Geometry: see drawing. Coordinates: mm, zero at the bounding-box minimum. A direction names the side the tool comes from. Round coordinates to 2 decimals unless told otherwise and drop trailing zeros. Loops run counter-clockwise (first coordinate to the right, second up) from the corner with the lowest first, then second, coordinate; pieces in that order, holes last. Notation, with made-up numbers: (84, 19.5) - (130, 19.5) arc R20 cw to (130, 28.5) - close; hole circle Ø6 at (40, 3.5). An arc over 180 degrees is marked (long way). Return JSON: item names as keys, results as strings. Group by question number.
1. Section A-A on y = 45. Return loops of the section in (x, z).
2. Section C-C on x = 20. Return loops of the section in (y, z) (1 decimal).
3. Draft query along X for the marked faces 1, 2 and 3. Return one class per face: +X half, -X half, draft (parallel to the pull), parting line (faces both ways), or undercut.
4. First-contact query: pin 1 Ø1.5 at (y, z) = (22.5, 1.5) entering from +X; pin 2 Ø1.5 at (y, z) = (26, 2) entering from -X. Flat tips, straight axial feed; report the tip coordinate or a pass-through.
5. Set-up query: the marked faces 4 and 5. Return all of +Z, -Z, +X, -X, +Y, -Y with unobstructed straight access to the full face (end or side cutting, diameter ignored); none if empty.
6. Material intervals for probe 1 along Y at (x, z) = (5, 1.5); probe 2 along Y at (x, z) = (26, 2.2) (1 decimal), sorted ascending.
7. Section B-B on x = 25. Return loops of the section in (y, z).
8. Section D-D on y = 34.5. Return loops of the section in (x, z) (1 decimal).
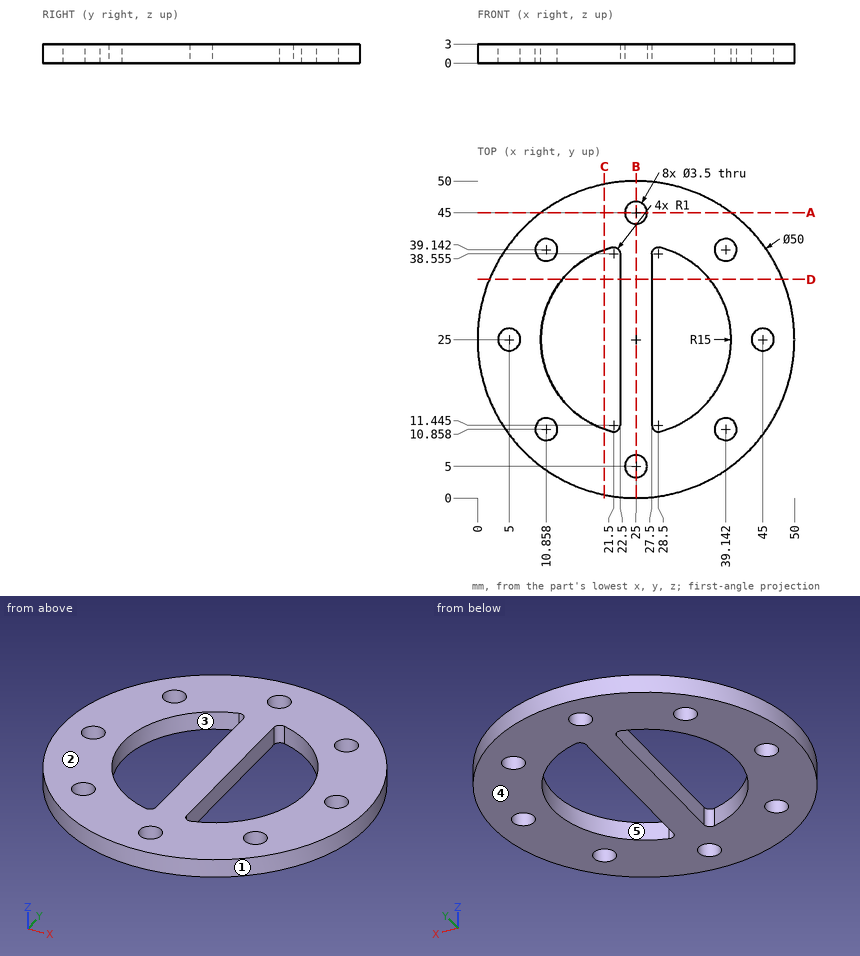
Taken from the geometry:
{
 "1": {"outline": "(10, 0) - (23.25, 0) - (23.25, 3) - (10, 3) - close; (26.75, 0) - (40, 0) - (40, 3) - (26.75, 3) - close"},
 "2": {"outline": "(0.5, 0) - (10.9, 0) - (10.9, 3) - (0.5, 3) - close; (39.1, 0) - (49.5, 0) - (49.5, 3) - (39.1, 3) - close"},
 "3": {"face 1": "parting line", "face 2": "draft", "face 3": "undercut"},
 "4": {"pin 1": "x = 49.94", "pin 2": "x = 0"},
 "5": {"face 4": "-Z, +X, -X, +Y, -Y", "face 5": "+Z, -Z"},
 "6": {"probe 1": "10 to 23.25, 26.75 to 40", "probe 2": "0 to 3.6, 6.4 to 43.6, 46.4 to 50"},
 "7": {"outline": "(0, 0) - (3.25, 0) - (3.25, 3) - (0, 3) - close; (6.75, 0) - (43.25, 0) - (43.25, 3) - (6.75, 3) - close; (46.75, 0) - (50, 0) - (50, 3) - (46.75, 3) - close"},
 "8": {"outline": "(1.9, 0) - (13.4, 0) - (13.4, 3) - (1.9, 3) - close; (22.5, 0) - (27.5, 0) - (27.5, 3) - (22.5, 3) - close; (36.6, 0) - (48.1, 0) - (48.1, 3) - (36.6, 3) - close"}
}
